The listing builds one solid part. Answer for the finished solid, in the listing's coordinates (mm). Round coordinates to 2 decimals unless told otherwise and drop trailing zeros. Loops run counter-clockwise (first coordinate to the right, second up) from the corner with the lowest first, then second, coordinate; pieces in that order, holes last. Notation, with made-up numbers: M -25.75,-27 L 22.25,-27 A10 ccw 22.25,-8 Z; hole C -33,36 d7. An arc over 180 degrees is marked long. Put each result on its own line as item: value. Start each with the question number.
(1) Section D-D, the plane z = -2.5 is taken. Determine the outline of the cut face in (x, y).
(2) Flat-ended cylindrical pins translate along their axes: P1, Ø5.5, axis at x = 4, y = -3.5, coming from the -Z side; P2, Ø2, axis at x = 0, z = -2, coming from the +Y side. Find the tip coordinate at first contact, or state that the pin passes through.
(3) Determine the mould class of faces 1 (the face through (2.066, -1.952, 0.74)), 2 (the face through (0, 0, 1.5)), 3 (the face through (-1.172, 8.923, 0.74)), 4 (the face through (0.536, -2.281, -0.986)) for opening direction Y: released by +Y, released by -Y, zero draft, split by the parting line, or undercut.
(4) Section A-A, the plane y = 0 is taken. Determine the outline of the cut face in (x, z).
(5) Section B-B, the plane x = 2.5 is taken. Determine the outline of the cut face in (y, z), then the cut area to 3 significant figures.
(6) Section C-C, the plane z = 0.45 is taken. Determine the outline of the cut face in (x, y), then the cut area to 3 significant figures.
(7) Straight lines are drawn through the part: line 1 (Y direction, x = 0, z = -1.75); line 2 (Z direction, x = -3.75, y = 8); line 3 (Y direction, x = 2.5, z = 0.8). For each, find the intervals that lie inside material, in ascending order.
```python
from build123d import *

# Parameters (mm, degrees)
SKETCH_2_R      = 9
SKETCH_2_R_2    = 2
EXTRUDE_1_DEPTH = 1.5
SKETCH_2_3_R    = 1
EXTRUDE_3_DEPTH = 3
FILLET_1_R      = 1


with BuildPart() as part:
    # 草图2 → 凸台-拉伸1 (new body)
    with BuildSketch(Plane.XY):
        Circle(SKETCH_2_R)
        with Locations((2.5, 0)):
            Circle(SKETCH_2_R_2, mode=Mode.SUBTRACT)
    extrude(amount=EXTRUDE_1_DEPTH)

    # 草图2<3> → 凸台-拉伸3 (add)
    with BuildSketch(Plane.XY):
        with Locations((-0.001510054, -3.123707411)):
            Circle(SKETCH_2_3_R)
        with Locations((-0.001510054, 3.123707411)):
            Circle(SKETCH_2_3_R)
    extrude(amount=-EXTRUDE_3_DEPTH)

    # 圆角1
    fillet_1_edges = [part.edges().sort_by_distance(p)[0] for p in [
        (-1.001510054, 3.123707411, -3),
        (-1.001510054, -3.123707411, -3),
    ]]
    fillet(fillet_1_edges, radius=FILLET_1_R)


solid = part.part
```
Recorded:
1. outline: C 0,-3.12 d1.73; C 0,3.12 d1.73
2. P1: stops at z = 0
2. P2: stops at y = 4.12
3. face 1: undercut
3. face 2: zero draft
3. face 3: split by the parting line
3. face 4: undercut
4. outline: M -9,0 L 0.5,0 L 0.5,1.5 L -9,1.5 Z; M 4.5,0 L 9,0 L 9,1.5 L 4.5,1.5 Z
5. outline: M -8.65,0 L -2,0 L -2,1.5 L -8.65,1.5 Z; M 2,0 L 8.65,0 L 8.65,1.5 L 2,1.5 Z
5. area: 19.9 mm²
6. outline: C 0,0 d18; hole C 2.5,0 d4
6. area: 242 mm²
7. line 1: y = -4.12 to -2.12, 2.12 to 4.12
7. line 2: z = 0 to 1.5
7. line 3: y = -8.65 to -2, 2 to 8.65
